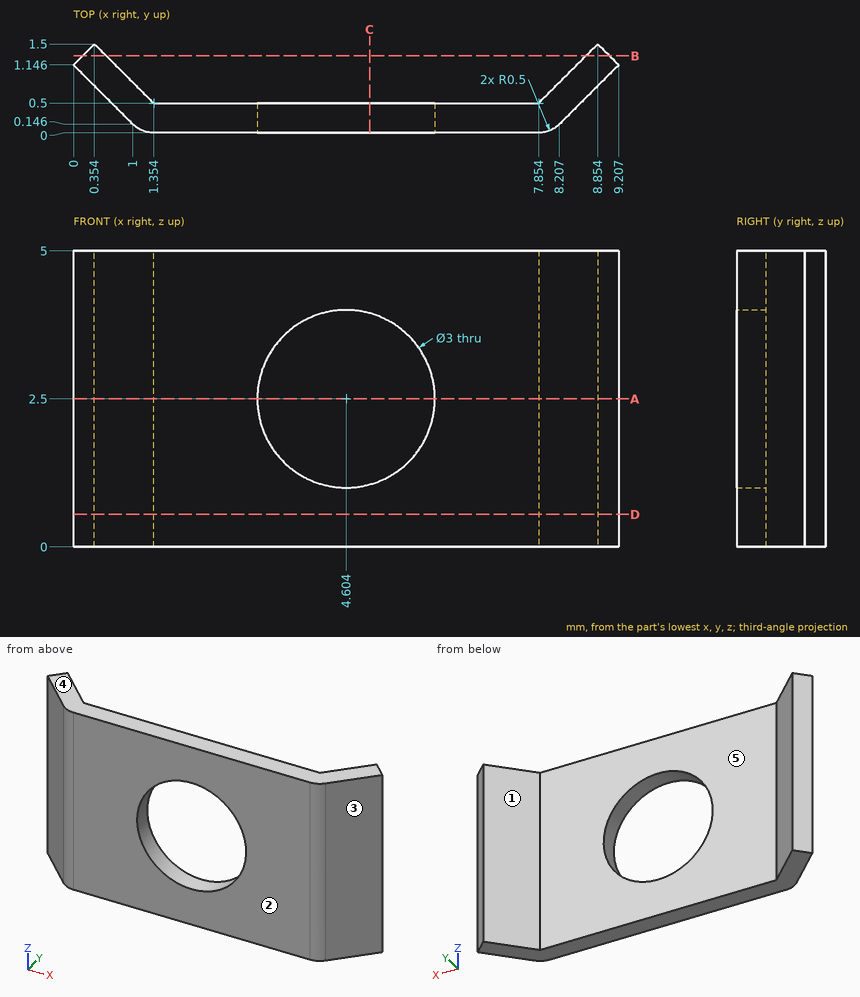
Verification items for this drawing (mm, ordinates from the low corner). A direction names the side the tool comes from. Coordinates: 2 decimals unless noted, no trailing zeros. Loops run counter-clockwise (first coordinate to the right, second up) from the corner with the lowest first, then second, coordinate; pieces in that order, holes last.
Item 1: Release check for a two-part mould opening along X. For the marked faces 1, 2 and 3 record: released by +X, released by -X, zero draft, split by the parting line, or undercut.
Item 2: Go/stop test with a flat-tipped pin: pin 1 Ø3 at (x, z) = (6.5, 1.5) entering from +Y (1 decimal). Record where the tip stops, or that it passes through.
Item 3: Sectioned sample at A-A, the plane z = 2.5. Record the boundary of the cut face in (x, y).
Item 4: Thickness scan on line 1 (Y direction, x = 1.75, z = 0.55); line 2 (X direction, y = 0.6, z = 2.75) (1 decimal); line 3 (X direction, y = 0.3, z = 2.5) (1 decimal). Record the ranges inside material, lowest first.
Item 5: Sectioned sample at B-B, the plane y = 1.3. Record the boundary of the cut face in (x, z).
Item 6: Sectioned sample at C-C, the plane x = 5. Record the boundary of the cut face in (y, z).
Item 7: Sectioned sample at D-D, the plane z = 0.55. Record the boundary of the cut face in (x, y).
Item 8: Access from +Z, -Z, +X, -X, +Y, -Y to the whole of each face (thin tool, end or side, straight path). Record for the marked faces 4 and 5.
Check result:
1. face 1: undercut
1. face 2: zero draft
1. face 3: released by +X
2. pin 1: stops at y = 0.6
3. outline: (0, 1.15) - (1, 0.15) arc R0.5 ccw to (1.35, 0) - (3.1, 0) - (3.1, 0.5) - (1.35, 0.5) - (0.35, 1.5) - close; (6.1, 0) - (7.85, 0) arc R0.5 ccw to (8.21, 0.15) - (9.21, 1.15) - (8.85, 1.5) - (7.85, 0.5) - (6.1, 0.5) - close
4. line 1: y = 0 to 0.5
4. line 2: x = 0.5 to 1.3, 8 to 8.7
4. line 3: x = 0.8 to 3.1, 6.1 to 8.4
5. outline: (0.15, 0) - (0.55, 0) - (0.55, 5) - (0.15, 5) - close; (8.65, 0) - (9.05, 0) - (9.05, 5) - (8.65, 5) - close
6. outline: (0, 0) - (0.5, 0) - (0.5, 1.05) - (0, 1.05) - close; (0, 3.95) - (0.5, 3.95) - (0.5, 5) - (0, 5) - close
7. outline: (0, 1.15) - (1, 0.15) arc R0.5 ccw to (1.35, 0) - (7.85, 0) arc R0.5 ccw to (8.21, 0.15) - (9.21, 1.15) - (8.85, 1.5) - (7.85, 0.5) - (1.35, 0.5) - (0.35, 1.5) - close
8. face 4: +Z, +X, -X, +Y, -Y
8. face 5: +Z, -Z, +Y
